```python
from build123d import *

# Parameters (mm, degrees)
F4_R = 3


with BuildPart() as f2:
    # F1 (on Front) → F2 (revolve)
    with BuildSketch(Plane.XZ):
        with BuildLine():
            Line((8, 10), (8, 0))
            Line((8, 0), (8.5, 0))
            Line((8.5, 0), (8.5, 10))
            ThreePointArc((8.5, 10), (8.3535533906, 10.3535533906), (8, 10.5))
            Line((8, 10.5), (0, 10.5))
            Line((0, 10.5), (0, 10))
            Line((0, 10), (8, 10))
        make_face()
    revolve(axis=Axis((0, 0, 0), (0, 0, 1)))

    # F5: sweep along a path in F3
    with BuildLine(Plane.YZ) as f5_path:
        Line((-53, 5.2680876106), (-8, 5.2680876106))
    # F4 (on Front) → F5 (sweep)
    with BuildSketch(Plane.XZ):
        with Locations((0, 5.3068501875)):
            Circle(F4_R)
    sweep(path=f5_path.line)


solid = f2.part
```
Geometry: final body of the model. Coordinates: model frame, mm. A direction names the side the tool comes from. Round coordinates to 2 decimals unless told otherwise and drop trailing zeros. Write each loop counter-clockwise with the first axis right and the second up, starting at its lowest first coordinate (ties: lowest second). Pieces come first, ordered by that corner, then holes. Notation, with made-up numbers: (-39, 6.5) -> (-26, 6.5) arc R8 ccw to (-26, 16.5) -> close; hole circle Ø2 at (37.25, -9.75). An arc over 180 degrees is marked (long way). Use CSV: the item, a comma, the result in double quotes. Start each with the question number.
Q1. First-contact query: pin 1 Ø5 at (x, y) = (0, -0.5) entering from -Z; pin 2 Ø3 at (y, z) = (-33, 3) entering from +X; pin 3 Ø4 at (x, z) = (-5, 8.5) entering from +Y. Flat tips, straight axial feed; report the tip coordinate or a pass-through.
Q2. Section A-A (z = 3.5). Return loops of the section in (x, y).
Q3. Line query: L1, parallel to Y at x = 0, z = 6.25; L2, parallel to X at y = -6, z = 3.5; L3, parallel to X at y = 0.5, z = 6.25. Output: solid intervals per line, ascending.
Q4. Reachability of faces 1 (the face through (-0.65, -3.946, 8.236)), 2 (the face through (0, -45, 5)), 3 (the face through (-0.391, -26.217, 2.332)) from +Z, -Z, +X, -X, +Y, -Y: full face, straight path, thin tool, end or side. Return the list, or none.
Q5. Pull-direction query (Z, two-part tool) for faces 4 (the face through (0, 0, 10)), 5 (the face through (0, 0, 5)), 6 (the face through (0, 0, 10.5)); classes: pulls with the +Z half, pulls with the -Z half, needs draft (parallel to the pull), parting line crosses it, or undercut.
Q6. Section D-D (z = 6). Return loops of the section in (x, y).
Q7. Section C-C (y = -18). Return loops of the section in (x, z).
Q8. Section B-B (x = 0). Return loops of the section in (y, z), plus the area to 3 significant figures.
Result sheet:
1,pin 1,"z = 2.31"
1,pin 2,"x = 2.89"
1,pin 3,"y = 7.95"
2,outline,"(-2.39, -45) -> (2.39, -45) -> (2.39, -8.16) arc R8.5 ccw (long way) to (-2.39, -8.16) -> close; hole (-2.39, -7.63) -> (-2.39, 0) -> (2.39, 0) -> (2.39, -7.63) arc R8 ccw (long way) to start"
3,L1,"-45 to 0, 8 to 8.5"
3,L2,"-6.02 to -5.29, -2.39 to 2.39, 5.29 to 6.02"
3,L3,"-8.49 to -7.98, 7.98 to 8.49"
4,face 1,"none"
4,face 2,"+Z, -Z, +X, -X, -Y"
4,face 3,"-Y"
5,face 4,"undercut"
5,face 5,"needs draft"
5,face 6,"pulls with the +Z half"
6,outline,"(-2.92, -45) -> (2.92, -45) -> (2.92, -7.98) arc R8.5 ccw (long way) to (-2.92, -7.98) -> close; hole (-2.92, -7.45) -> (-2.92, 0) -> (2.92, 0) -> (2.92, -7.45) arc R8 ccw (long way) to start"
7,outline,"circle Ø6 at (0, 5.31)"
8,outline,"(-45, 2.31) -> (-8.5, 2.31) -> (-8.5, 0) -> (-8, 0) -> (-8, 2.31) -> (0, 2.31) -> (0, 8.31) -> (-8, 8.31) -> (-8, 10) -> (8, 10) -> (8, 0) -> (8.5, 0) -> (8.5, 10) arc R0.5 ccw to (8, 10.5) -> (-8, 10.5) arc R0.5 ccw to (-8.5, 10) -> (-8.5, 8.31) -> (-45, 8.31) -> close"
8,area,"285 mm²"
